```python
from build123d import *

# Parameters (mm, degrees)
F1_DEPTH = 0.5
F3_DEPTH = 0.501
F5_DEPTH = 0.501


with BuildPart() as f1:
    # F0 (on Top) → F1 (new body)
    with BuildSketch(Plane.XY):
        Polygon((6.25, -10.825318), (12.5, 0), (6.25, 10.825318), (-6.25, 10.825318), (-12.5, 0), (-6.25, -10.825318), align=None)
    extrude(amount=F1_DEPTH)

    # F2 (on face) → F3 (cut, through all)
    with BuildSketch(Plane.XY.offset(0.5)):
        with BuildLine():
            ThreePointArc((0.85, -10.825318), (0.674264, -10.401053), (0.25, -10.225318))
            Line((0.25, -10.225318), (-0.25, -10.225318))
            ThreePointArc((-0.25, -10.225318), (-0.674264, -10.401053), (-0.85, -10.825318))
            Line((-0.85, -10.825318), (0.85, -10.825318))
        make_face()
    extrude(amount=-F3_DEPTH, mode=Mode.SUBTRACT)

    # F4 (on face) → F5 (cut, through all)
    with BuildSketch(Plane.XY.offset(0.5)):
        Polygon((-6.25, 10.825318), (-12.5, 0), (12.5, 0), (6.25, 10.825318), align=None)
    extrude(amount=-F5_DEPTH, mode=Mode.SUBTRACT)


solid = f1.part
```
For this review, take the finished solid that the model builds, in its own axes (mm). Round coordinates to 2 decimals unless told otherwise and drop trailing zeros. Order: outer loops, then holes, each group sorted by start corner. A loop starts at its lowest first (then second) coordinate and runs counter-clockwise, first axis right, second up.
Q1. We need section B-B, the plane y = -2.5. Give the boundary of the cut face in (x, z).
Findings below:
outline: (-11.06, 0) - (11.06, 0) - (11.06, 0.5) - (-11.06, 0.5) - close
Q2. We need section A-A, the plane z = 0.3. Give the boundary of the cut face in (x, y), plus the area to 3 significant figures.
Findings below:
outline: (-12.5, 0) - (-6.25, -10.83) - (-0.85, -10.83) arc R0.6 cw to (-0.25, -10.23) - (0.25, -10.23) arc R0.6 cw to (0.85, -10.83) - (6.25, -10.83) - (12.5, 0) - close
area: 202 mm2
Q3. Wall thickness on line 1 (X direction, y = -1.5, z = 0.1); line 2 (X direction, y = -4, z = 0.45); line 3 (Y direction, x = -6.75, z = 0.4): over which ranges is each line inside the solid? List them lowest first.
Findings below:
line 1: x = -11.63 to 11.63
line 2: x = -10.19 to 10.19
line 3: y = -9.96 to 0
Q4. We need section C-C, the plane x = 7. Give the boundary of the cut face in (y, z).
Findings below:
outline: (-9.53, 0) - (0, 0) - (0, 0.5) - (-9.53, 0.5) - close
